```python
from build123d import *

# Parameters (mm, degrees)
EXTRUDE_1_DEPTH             = 11.5
FILLET_1_R                  = 0.3
FILLET_2_R                  = 2
HOLE_WIZARD_M63_D           = 5
HOLE_WIZARD_M63_CSINK_D     = 6.05
HOLE_WIZARD_M63_CSINK_ANGLE = 90


with BuildPart() as part:
    # Эскиз1 → Бобышка-Вытянуть1 (new body, symmetric)
    with BuildSketch(Plane.XY):
        with BuildLine():
            Line((-5, 0), (5, 0))
            Line((5, 0), (5, -0.8))
            Line((5, -0.8), (8, -0.8))
            Line((8, -0.8), (8, -1.6))
            ThreePointArc((8, -1.6), (5.309398779, -5.576969864), (1.5, -8.5))
            Line((1.5, -8.5), (-1.5, -8.5))
            ThreePointArc((-1.5, -8.5), (-5.309398779, -5.576969864), (-8, -1.6))
            Line((-8, -1.6), (-8, -0.8))
            Line((-8, -0.8), (-5, -0.8))
            Line((-5, -0.8), (-5, 0))
        make_face()
    extrude(amount=EXTRUDE_1_DEPTH, both=True)

    # Скругление1
    fillet_1_edges = [part.edges().sort_by_distance(p)[0] for p in [
        (8, -0.8, 0),
        (8, -1.6, 0),
        (-8, -1.6, 0),
        (-8, -0.8, 0),
        (-5, 0, 0),
        (5, 0, 0),
    ]]
    fillet(fillet_1_edges, radius=FILLET_1_R)

    # Скругление2
    fillet_2_edges = [part.edges().sort_by_distance(p)[0] for p in [
        (1.5, -8.5, 0),
        (-1.5, -8.5, 0),
    ]]
    fillet(fillet_2_edges, radius=FILLET_2_R)

    # Отверстие обработанное метчиком M63 (through all)
    with Locations(Plane(origin=(0, 0, 0), x_dir=(1, 0, 0), z_dir=(0, 1, 0))):
        with Locations((0, -4.5)):
            CounterSinkHole(HOLE_WIZARD_M63_D / 2, HOLE_WIZARD_M63_CSINK_D / 2, counter_sink_angle=HOLE_WIZARD_M63_CSINK_ANGLE)

    # Эскиз5 → Повернуть1 (revolve)
    with BuildSketch(Plane(origin=(0, 0, 0), x_dir=(0, 0, -1), z_dir=(1, 0, 0))):
        with BuildLine():
            Line((6.5, -4.3), (6.5, -9.3))
            ThreePointArc((6.5, -9.3), (4, -6.8), (6.5, -4.3))
        make_face()
    revolve(axis=Axis((0, -4.3, -6.5), (0, -1, 0)))


solid = part.part
```
Geometry check sheet. Reference: the model listing, model coordinates, mm. A direction names the side the tool comes from. Coordinates: 2 decimals unless noted, no trailing zeros. Order: outer loops, then holes, each group sorted by start corner. A loop starts at its lowest first (then second) coordinate and runs counter-clockwise, first axis right, second up.
Item 1: Depth check by flat-ended pin: pin 1 (2 mm diameter, centred on x = 0, z = -0.5, fed in from -Y); pin 2 (4 mm diameter, centred on y = -4, z = 6, fed in from -X); pin 3 (1.4 mm diameter, centred on x = -6, z = -1, fed in from +Y). Enter the tip coordinate at first touch or a pass-through.
Item 2: Section check B-B (y = -5). Enter the section's corners in (x, z), plus the area to 3 significant figures.
Item 3: Scan lines: line 1 along Z through (x, y) = (0, -3.5); line 2 along X through (y, z) = (-5.5, 3.5); line 3 along Z through (x, y) = (1, -2.25). Record each from-to range of solid material in increasing order.
Item 4: Section check D-D (y = -3.25). Enter the section's corners in (x, z).
Item 5: Section check A-A (x = 0). Enter the section's corners in (y, z) (3 decimals).
Item 6: Tool access check on faces 1 (the flat face through (0, -8.5, 9)), 2 (the cylindrical face through (1.509, -8.428, -9.786)), 3 (the cylindrical face through (1.509, -8.428, 8.718)). Record the directions out of +Z, -Z, +X, -X, +Y, -Y that give a thin tool (end or side, any length) a straight path to the whole face; none if there is none.
Item 7: Mould release check, pull along X, two halves, no side actions. Record for faces 4 (the cylindrical face through (2.5, -4.6, 4.4)), 5 (the cylindrical face through (-1.509, -8.428, 8.718)), 6 (the flat face through (0, -8.5, -10)): released by +X, released by -X, zero draft, split by the parting line, or undercut.
Check sheet entries:
1. pin 1: stops at y = -8.5
1. pin 2: stops at x = -7.81
1. pin 3: stops at y = -0.8
2. outline: (-5.83, -11.5) - (5.83, -11.5) - (5.83, 11.5) - (-5.83, 11.5) - close; hole circle Ø5 at (0, 4.5)
2. area: 248 mm2
3. line 1: z = -11.5 to 2, 7 to 11.5
3. line 2: x = -5.38 to -2.29, 2.29 to 5.38
3. line 3: z = -11.5 to 2.21, 6.79 to 11.5
4. outline: (-7.11, -11.5) - (7.11, -11.5) - (7.11, 11.5) - (-7.11, 11.5) - close; hole circle Ø5 at (0, 4.5)
5. outline: (-8.5, -11.5) - (0, -11.5) - (0, 1.475) - (-0.525, 2) - (-8.5, 2) - (-8.5, -4.667) arc R2.5 ccw to (-8.5, -8.333) - close; (-8.5, 7) - (-0.525, 7) - (0, 7.525) - (0, 11.5) - (-8.5, 11.5) - close
6. face 1: +Z, +X, -X, -Y
6. face 2: -Z, +X, -Y
6. face 3: +Z, +X, -Y
7. face 4: undercut
7. face 5: released by -X
7. face 6: zero draft
